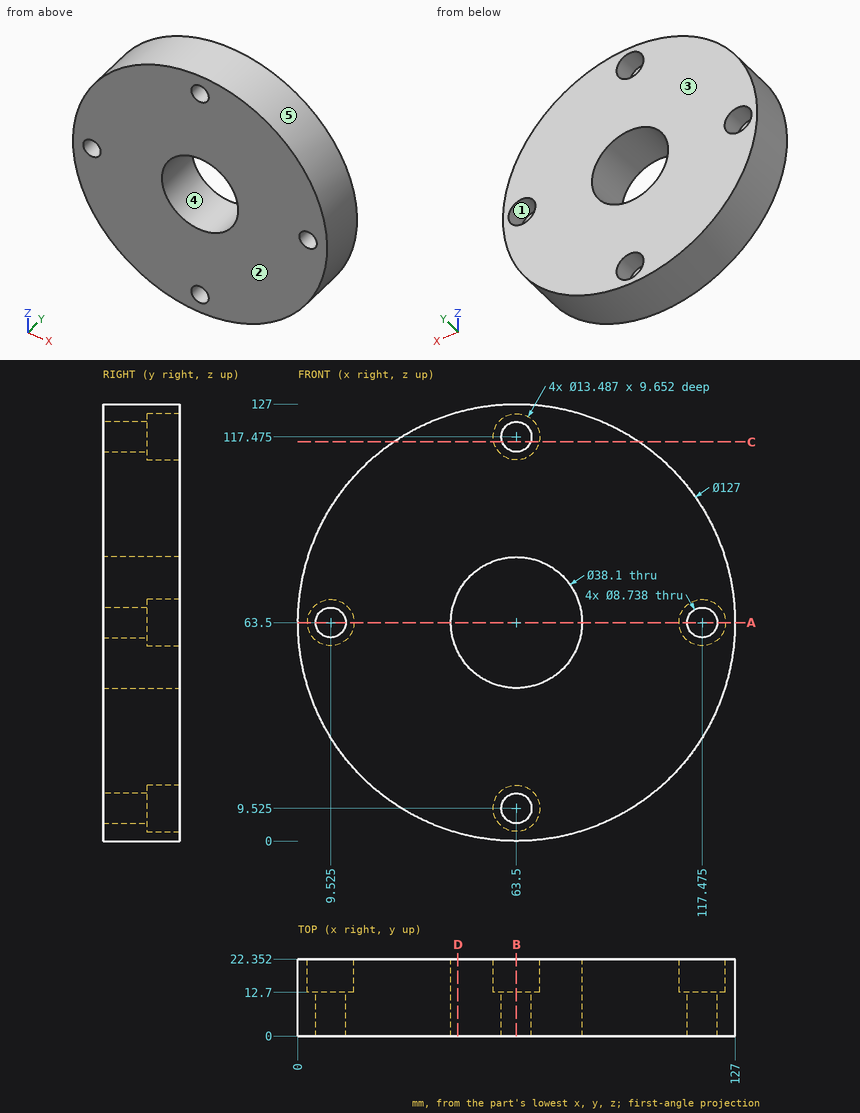
Input: dimensioned drawing with shaded views. Units: mm. Origin: part minimum x, y, z. A direction names the side the tool comes from. Give positions to 0.01 mm unless a question says otherwise; leave off trailing zeros. Loops run counter-clockwise (first coordinate to the right, second up) from the corner with the lowest first, then second, coordinate; pieces in that order, holes last. Notation, with made-up numbers: (38.25, -32.5) -> (61.25, -32.5) arc R26 ccw to (61.25, -0.5) -> close; hole circle Ø6 at (72.25, 15). An arc over 180 degrees is marked (long way). Use a Markdown table: item, result. Add a question column.
1) Pull-direction query (Z, two-part tool) for the marked faces 3, 4 and 5; classes: +Z half, -Z half, draft (parallel to the pull), parting line (faces both ways), or undercut.
2) Line query: line 1 along X through (y, z) = (14.5, 69) (1 decimal); line 2 along X through (y, z) = (19, 63.5); line 3 along X through (y, z) = (12.25, 118) (1 decimal). Output: solid intervals per line, ascending. Write a range as [from, to].
3) Reachability of the marked faces 1 and 2 from +Z, -Z, +X, -X, +Y, -Y: full face, straight path, thin tool, end or side. Return the list, or none.
4) Section query B-B, the plane x = 63.5. Return the cut outline in (y, z).
5) Section query A-A, the plane z = 63.5. Return the cut outline in (x, y).
6) First-contact query: pin 1 (15.5 mm diameter, centred on x = 63.5, z = 117.475, fed in from +Y); pin 2 (3 mm diameter, centred on x = 17, y = 11.5, fed in from +Z); pin 3 (10 mm diameter, centred on x = 9.525, z = 63.5, fed in from +Y); pin 4 (5 mm diameter, centred on y = 5, z = 82.5, fed in from +X). Flat tips, straight axial feed; report the tip coordinate or a pass-through.
7) Section query C-C, the plane z = 116. Return the cut outline in (x, y).
8) Section query D-D, the plane x = 46.5. Return the cut outline in (y, z).
Numbers:
| question | item | result |
|---|---|---|
| 1 | face 3 | draft |
| 1 | face 4 | undercut |
| 1 | face 5 | parting line |
| 2 | line 1 | x = [0.2, 5.6], [13.4, 45.3], [81.7, 113.6], [121.4, 126.8] |
| 2 | line 2 | x = [0, 2.78], [16.27, 44.45], [82.55, 110.73], [124.22, 127] |
| 2 | line 3 | x = [30.9, 59.2], [67.8, 96.1] |
| 3 | face 1 | +Y |
| 3 | face 2 | +Z, -Z, +X, -X, -Y |
| 4 | outline | (0, 0) -> (22.35, 0) -> (22.35, 2.78) -> (12.7, 2.78) -> (12.7, 5.16) -> (0, 5.16) -> close; (0, 13.89) -> (12.7, 13.89) -> (12.7, 16.27) -> (22.35, 16.27) -> (22.35, 44.45) -> (0, 44.45) -> close; (0, 82.55) -> (22.35, 82.55) -> (22.35, 110.73) -> (12.7, 110.73) -> (12.7, 113.11) -> (0, 113.11) -> close; (0, 121.84) -> (12.7, 121.84) -> (12.7, 124.22) -> (22.35, 124.22) -> (22.35, 127) -> (0, 127) -> close |
| 5 | outline | (0, 0) -> (5.16, 0) -> (5.16, 12.7) -> (2.78, 12.7) -> (2.78, 22.35) -> (0, 22.35) -> close; (13.89, 0) -> (44.45, 0) -> (44.45, 22.35) -> (16.27, 22.35) -> (16.27, 12.7) -> (13.89, 12.7) -> close; (82.55, 0) -> (113.11, 0) -> (113.11, 12.7) -> (110.73, 12.7) -> (110.73, 22.35) -> (82.55, 22.35) -> close; (121.84, 0) -> (127, 0) -> (127, 22.35) -> (124.22, 22.35) -> (124.22, 12.7) -> (121.84, 12.7) -> close |
| 6 | pin 1 | stops at y = 22.35 |
| 6 | pin 2 | stops at z = 108.3 |
| 6 | pin 3 | stops at y = 12.7 |
| 6 | pin 4 | stops at x = 124.82 |
| 7 | outline | (27.78, 0) -> (59.39, 0) -> (59.39, 12.7) -> (56.92, 12.7) -> (56.92, 22.35) -> (27.78, 22.35) -> close; (67.61, 0) -> (99.22, 0) -> (99.22, 22.35) -> (70.08, 22.35) -> (70.08, 12.7) -> (67.61, 12.7) -> close |
| 8 | outline | (0, 2.32) -> (22.35, 2.32) -> (22.35, 54.9) -> (0, 54.9) -> close; (0, 72.1) -> (22.35, 72.1) -> (22.35, 124.68) -> (0, 124.68) -> close |
